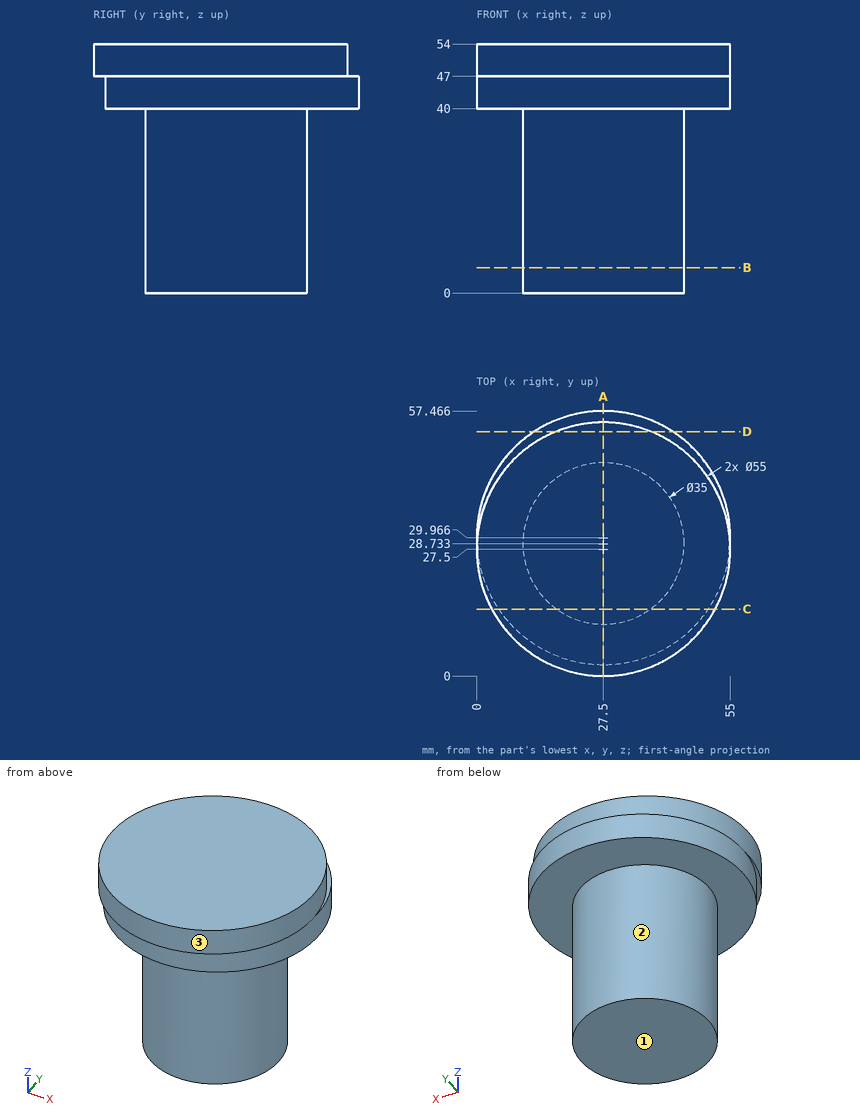
Input: dimensioned drawing with shaded views. Units: mm. Origin: part minimum x, y, z. A direction names the side the tool comes from. Give positions to 0.01 mm unless a question says otherwise; leave off trailing zeros. Write each loop counter-clockwise with the first axis right and the second up, starting at its lowest first coordinate (ties: lowest second). Pieces come first, ordered by that corner, then holes.
1. Line query: probe 1 along Z at (x, y) = (33, 4.5); probe 2 along Z at (x, y) = (48, 47); probe 3 along X at (y, z) = (23, 7). Output: solid intervals per line, ascending.
2. Section query D-D, the plane y = 53. Return loops of the section in (x, z).
3. Section query B-B, the plane z = 5.5. Return loops of the section in (x, y).
4. Section query A-A, the plane x = 27.5. Return loops of the section in (y, z), then the cut area to 3 significant figures.
5. Reachability of the marked faces 1, 2 and 3 from +Z, -Z, +X, -X, +Y, -Y: full face, straight path, thin tool, end or side. Return the list, or none.
6. Section query C-C, the plane y = 14.5. Return loops of the section in (x, z).
7. Pin query (flat end, axial travel): P1, Ø10, axis at y = 36.5, z = 37.5, coming from the +X side; P2, Ø3, axis at x = 39.5, z = 5.5, coming from the +Y side; P3, Ø2, axis at y = 29.5, z = 34, coming from the -X side; P4, Ø23, axis at x = 24, y = 16, coming from the -Z side. Return the tip coordinate at first contact, or that it passes through.
Computed:
1. probe 1: z = 40 to 54
1. probe 2: z = 40 to 47
1. probe 3: x = 10.97 to 44.03
2. outline: (12.48, 40) - (42.52, 40) - (42.52, 47) - (37.8, 47) - (37.8, 54) - (17.2, 54) - (17.2, 47) - (12.48, 47) - close
3. outline: circle Ø35 at (27.5, 28.73)
4. outline: (0, 47) - (2.47, 47) - (2.47, 40) - (11.23, 40) - (11.23, 0) - (46.23, 0) - (46.23, 40) - (57.47, 40) - (57.47, 47) - (55, 47) - (55, 54) - (0, 54) - close
4. area: 2,170 mm2
5. face 1: -Z, +X, -X, +Y, -Y
5. face 2: -Z
5. face 3: +Z
6. outline: (3.27, 47) - (4.76, 47) - (4.76, 40) - (17.32, 40) - (17.32, 0) - (37.68, 0) - (37.68, 40) - (50.24, 40) - (50.24, 47) - (51.73, 47) - (51.73, 54) - (3.27, 54) - close
7. P1: stops at x = 54.91
7. P2: stops at y = 42.73
7. P3: stops at x = 10
7. P4: stops at z = 0
